Geometry: final body of the model. Coordinates: model frame, mm. A direction names the side the tool comes from. Round coordinates to 2 decimals unless told otherwise and drop trailing zeros. Loops run counter-clockwise (first coordinate to the right, second up) from the corner with the lowest first, then second, coordinate; pieces in that order, holes last. Notation, with made-up numbers: (68.25, 87) -> (93.25, 87) arc R36 cw to (93.25, 122) -> close; hole circle Ø2 at (51, 65.25). An arc over 180 degrees is marked (long way). Answer in a Markdown table with one row per item.
```python
from build123d import *

# Parameters (mm, degrees)
SKETCH1_W           = 118
SKETCH1_H           = 52
SKETCH1_R           = 2
BOSS_EXTRUDE1_DEPTH = 2.5
BOSS_EXTRUDE2_DEPTH = 1.7


with BuildPart() as part:
    # Sketch1 → Boss-Extrude1 (new body)
    with BuildSketch(Plane.XY):
        with Locations((39.179079988, -106.041481737)):
            Rectangle(SKETCH1_W, SKETCH1_H)
        with Locations((-16.638939496, -128.859501222)):
            Circle(SKETCH1_R, mode=Mode.SUBTRACT)
        with Locations((94.997099473, -128.859501222)):
            Circle(SKETCH1_R, mode=Mode.SUBTRACT)
        with Locations((94.997099473, -83.223462252)):
            Circle(SKETCH1_R, mode=Mode.SUBTRACT)
        with Locations((-16.638939496, -83.223462252)):
            Circle(SKETCH1_R, mode=Mode.SUBTRACT)
    extrude(amount=BOSS_EXTRUDE1_DEPTH)

    # Sketch2 → Boss-Extrude2 (add)
    with BuildSketch(Plane.XY.offset(2.5)):
        Polygon((14.823144888, -94.914102462), (16.746221811, -94.914102462), (23.412888478, -110.67532041), (30.079555144, -94.914102462), (32.002632067, -94.914102462), (23.541093606, -114.914102462), (23.284683349, -114.914102462), align=None)
        Polygon((38.048305144, -94.914102462), (41.746221811, -94.914102462), (41.746221811, -114.914102462), (39.951350016, -114.914102462), (39.951350016, -96.965384513), (36.874426939, -96.965384513), align=None)
    extrude(amount=BOSS_EXTRUDE2_DEPTH)


solid = part.part
```
Item 1: Mould query, pull axis Y, two halves, no side actions, for faces 1 (the flat face through (98.179, -106, 1)), 2 (the cylindrical face through (-16.9, -81.24, 1.23)), 3 (the flat face through (20.03, -102.68, 3.34)). Classes: released by +Y, released by -Y, zero draft, split by the parting line, or undercut.
Ans:
| item | result |
|---|---|
| face 1 | zero draft |
| face 2 | undercut |
| face 3 | released by +Y |
Item 2: First-contact query: P1, Ø4.5, axis at x = 95, y = -128.86, coming from the +Z side; P2, Ø0.5, axis at x = 39.5, z = 3.5, coming from the +Y side; P3, Ø3, axis at x = -16.64, y = -128.86, coming from the -Z side; P4, Ø1.9, axis at y = -102, z = 3.5, coming from the +X side. Flat tips, straight axial feed; report the tip coordinate or a pass-through.
Ans:
| item | result |
|---|---|
| P1 | z = 2.5 |
| P2 | y = -94.91 |
| P3 | through |
| P4 | x = 41.75 |
Item 3: Section query A-A, the plane y = -100. Output: boundary loops of the cut face in (x, z).
Ans:
| item | result |
|---|---|
| outline | (-19.82, 0) -> (98.18, 0) -> (98.18, 2.5) -> (41.75, 2.5) -> (41.75, 4.2) -> (39.95, 4.2) -> (39.95, 2.5) -> (29.85, 2.5) -> (29.85, 4.2) -> (27.93, 4.2) -> (27.93, 2.5) -> (18.9, 2.5) -> (18.9, 4.2) -> (16.97, 4.2) -> (16.97, 2.5) -> (-19.82, 2.5) -> close |
Item 4: Section query C-C, the plane y = -92. Output: boundary loops of the cut face in (x, z), and give its area (3 significant figures).
Ans:
| item | result |
|---|---|
| outline | (-19.82, 0) -> (98.18, 0) -> (98.18, 2.5) -> (-19.82, 2.5) -> close |
| area | 295 mm2 |
Item 5: Set-up query: faces 4 (the cylindrical face through (96.072, -81.537, 1.232)), 5 (the flat face through (19.11, -105.05, 3.34)), 6 (the flat face through (27.831, -104.774, 3.338)), 7 (the flat face through (26.7, -102.9, 3.3)). Return all of +Z, -Z, +X, -X, +Y, -Y with unobstructed straight access to the full face (end or side cutting, diameter ignored); none if empty.
Ans:
| item | result |
|---|---|
| face 4 | +Z, -Z |
| face 5 | +Z, -X, -Y |
| face 6 | +Z, -Y |
| face 7 | +Z, +Y |
Item 6: Section query D-D, the plane x = 43.5. Output: boundary loops of the cut face in (y, z).
Ans:
| item | result |
|---|---|
| outline | (-132.04, 0) -> (-80.04, 0) -> (-80.04, 2.5) -> (-132.04, 2.5) -> close |
Item 7: Ray query, L1, parallel to X at y = -99.5, z = 3.9; L2, parallel to X at y = -109, z = 2.7; L3, parallel to Z at x = 56, y = -89.5. Return the intervals inside material, ascending.
Ans:
| item | result |
|---|---|
| L1 | 16.76 to 18.69, 28.14 to 30.06, 39.95 to 41.75 |
| L2 | 20.78 to 22.7, 24.12 to 26.04, 39.95 to 41.75 |
| L3 | 0 to 2.5 |
Item 8: Section query B-B, the plane x = 27. Output: boundary loops of the cut face in (y, z).
Ans:
| item | result |
|---|---|
| outline | (-132.04, 0) -> (-80.04, 0) -> (-80.04, 2.5) -> (-102.19, 2.5) -> (-102.19, 4.2) -> (-106.74, 4.2) -> (-106.74, 2.5) -> (-132.04, 2.5) -> close |
